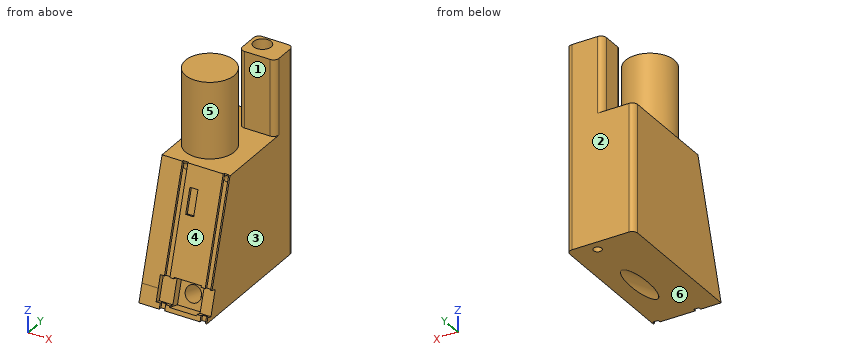
from build123d import *

# Parameters (mm, degrees)
SKETCH_1_W               = 25
SKETCH_1_H               = 60
EXTRUDE_1_DEPTH          = 75
SKETCH_3_R               = 9
CUT_EXTRUDE_1_DEPTH      = 58.142366069
SKETCH_4_R               = 3.25
CUT_EXTRUDE_2_DEPTH      = 62.320877358
SKETCH_5_R               = 1.5
CUT_EXTRUDE_3_DEPTH      = 62.320877358
SKETCH_6_W               = 25
SKETCH_6_H               = 5
CUT_EXTRUDE_4_DEPTH      = 82.738913621
CUT_EXTRUDE_5_DEPTH      = 85.557672626
SKETCH_9_R               = 3
CUT_EXTRUDE_6_DEPTH      = 85.994924721
SKETCH_10_W              = 10
SKETCH_10_H              = 10
CUT_EXTRUDE_7_DEPTH      = 5
CUT_EXTRUDE_8_DEPTH      = 15
CUT_EXTRUDE_8_DEPTH_BACK = 5
SKETCH_12_R              = 1
CUT_EXTRUDE_9_DEPTH      = 10
SKETCH_14_W              = 2
SKETCH_14_H              = 1
CUT_EXTRUDE_10_DEPTH     = 49.16
SKETCH_15_W              = 2.940527474
SKETCH_15_H              = 9
CUT_EXTRUDE_11_DEPTH     = 1
FILLET_1_R               = 2


with BuildPart() as part:
    # Эскиз1 → Бобышка-Вытянуть1 (new body)
    with BuildSketch(Plane.XY):
        Rectangle(SKETCH_1_W, SKETCH_1_H)
    extrude(amount=EXTRUDE_1_DEPTH)

    # Эскиз3 → Вырез-Вытянуть1 (cut, through all)
    with BuildSketch(Plane.XY.offset(47)):
        Polygon((-12.5, -30), (12.5, -30), (12.5, 14.25), (-1, 14.25), (-1, 30), (-12.5, 30), align=None)
        with Locations(Location((-3, 0, 0), (0, 0, 180))):
            Circle(SKETCH_3_R, mode=Mode.SUBTRACT)
    extrude(amount=CUT_EXTRUDE_1_DEPTH, mode=Mode.SUBTRACT)

    # Эскиз4 → Вырез-Вытянуть2 (cut, through all)
    with BuildSketch(Plane.XY.offset(52)):
        with Locations((3.5, 21)):
            Circle(SKETCH_4_R)
    extrude(amount=CUT_EXTRUDE_2_DEPTH, mode=Mode.SUBTRACT)

    # Эскиз5 → Вырез-Вытянуть3 (cut, through all)
    with BuildSketch(Plane.XY.offset(52)):
        with Locations((3.5, 21)):
            Circle(SKETCH_5_R)
    extrude(amount=-CUT_EXTRUDE_3_DEPTH, mode=Mode.SUBTRACT)

    # Эскиз6 → Вырез-Вытянуть4 (cut, through all)
    with BuildSketch(Plane(origin=(0, 0, 0), x_dir=(-1, 0, 0), z_dir=(0, 0, -1))):
        with Locations((0, 27.5)):
            Rectangle(SKETCH_6_W, SKETCH_6_H)
    extrude(amount=-CUT_EXTRUDE_4_DEPTH, mode=Mode.SUBTRACT)

    # Эскиз8 → Вырез-Вытянуть5 (cut, through all)
    with BuildSketch(Plane(origin=(12.5, 0, 0), x_dir=(0, 0, -1), z_dir=(1, 0, 0))):
        Polygon((-6.266839037, -25.421365839), (-47, -13.294552658), (-47, -30), (0, -30), (0, -27.287088617), align=None)
    extrude(amount=-CUT_EXTRUDE_5_DEPTH, mode=Mode.SUBTRACT)

    # Эскиз9 → Вырез-Вытянуть6 (cut, through all)
    with BuildSketch(Plane(origin=(0, -25.065453583, 7.462324694), x_dir=(1, 0, 0), z_dir=(0, -0.9584273167859609, 0.2853367807319331))):
        with Locations(Location((3.5, -1.247340968, 0), (0, 0, 270))):
            Circle(SKETCH_9_R)
    extrude(amount=-CUT_EXTRUDE_6_DEPTH, mode=Mode.SUBTRACT)

    # Эскиз10 → Вырез-Вытянуть7 (cut)
    with BuildSketch(Plane(origin=(0, -25.065453583, 7.462324694), x_dir=(1, 0, 0), z_dir=(0, -0.9584273167859609, 0.2853367807319331))):
        with Locations((3.5, -1.247340968)):
            Rectangle(SKETCH_10_W, SKETCH_10_H)
    extrude(amount=-CUT_EXTRUDE_7_DEPTH, mode=Mode.SUBTRACT)

    # Эскиз11 → Вырез-Вытянуть8 (cut, two sides: drawn at the far end of the back side and taken through both)
    with BuildSketch(Plane(origin=(-1.5, 0, 0), x_dir=(0, 0, -1), z_dir=(1, 0, 0)).offset(-CUT_EXTRUDE_8_DEPTH_BACK)):
        Polygon((-10.579761962, -24.137350326), (-1.953916111, -26.705381353), (-1.38324255, -24.788526719), (-10.009088401, -22.220495692), align=None)
    extrude(amount=CUT_EXTRUDE_8_DEPTH + CUT_EXTRUDE_8_DEPTH_BACK, mode=Mode.SUBTRACT)

    # Эскиз12 → Вырез-Вытянуть9 (cut)
    with BuildSketch(Plane(origin=(0, -25.065453583, 7.462324694), x_dir=(1, 0, 0), z_dir=(0, -0.9584273167859609, 0.2853367807319331))):
        with Locations(Location((-4, 39.752659032, 0), (0, 0, 270))):
            Circle(SKETCH_12_R)
        with Locations(Location((11, 39.752659032, 0), (0, 0, 90))):
            Circle(SKETCH_12_R)
    extrude(amount=-CUT_EXTRUDE_9_DEPTH, mode=Mode.SUBTRACT)

    # Эскиз14 → Вырез-Вытянуть10 (cut)
    with BuildSketch(Plane(origin=(0, -55.116213781, 8.285107119), x_dir=(-1, 0, 0), z_dir=(0, 0.285336780731933, 0.9584273167859609))):
        with Locations((4, -29.536239553)):
            Rectangle(SKETCH_14_W, SKETCH_14_H)
        with Locations((-11, -29.536239553)):
            Rectangle(SKETCH_14_W, SKETCH_14_H)
    extrude(amount=CUT_EXTRUDE_10_DEPTH, mode=Mode.SUBTRACT)

    # Эскиз15 → Вырез-Вытянуть11 (cut)
    with BuildSketch(Plane(origin=(0, -25.065453583, 7.462324694), x_dir=(1, 0, 0), z_dir=(0, -0.9584273167859609, 0.2853367807319331))):
        with Locations((0.529736263, 29.252659032)):
            Rectangle(SKETCH_15_W, SKETCH_15_H)
    extrude(amount=-CUT_EXTRUDE_11_DEPTH, mode=Mode.SUBTRACT)

    # Скругление1
    fillet_1_edges = [part.edges().sort_by_distance(p)[0] for p in [
        (12.5, 14.25, 61),
        (-1, 14.25, 61),
        (-1, 25, 61),
        (-12.5, 25, 23.5),
        (12.5, 25, 37.5),
    ]]
    fillet(fillet_1_edges, radius=FILLET_1_R)


solid = part.part
Read the model definition and answer for the solid it produces. Units are mm, in the model's axes. Face numbers are marked on the shaded views. A direction names the side the tool comes from. Give positions to 0.01 mm unless a question says otherwise; leave off trailing zeros. Loops run counter-clockwise (first coordinate to the right, second up) from the corner with the lowest first, then second, coordinate; pieces in that order, holes last. Notation, with made-up numbers: (-21, 64) -> (24, 64) arc R18 ccw to (24, 94) -> close; hole circle Ø8 at (-23, -24). An arc over 180 degrees is marked (long way). Answer as CSV lines item,"result".
Item 1: Find section B-B on y = 21. Give the vertices of the cut face in (x, z), plus the area to 3 significant figures.
Returned:
outline,"(-12.5, 0) -> (2, 0) -> (2, 52) -> (0.25, 52) -> (0.25, 75) -> (-1, 75) -> (-1, 47) -> (-12.5, 47) -> close; (5, 0) -> (12.5, 0) -> (12.5, 75) -> (6.75, 75) -> (6.75, 52) -> (5, 52) -> close"
area,"1,250 mm²"
Item 2: For the marked faces 5 and 6, determine the directions among +Z, -Z, +X, -X, +Y, -Y from which every point of the face is accessible in a straight line to the end or side of a thin tool.
Returned:
face 5,"+Z"
face 6,"-Z, +X, -X, +Y, -Y"
Item 3: Consider line 1 (X direction, y = 21, z = 60.75); line 2 (Y direction, x = 3.5, z = 64.25); line 3 (Y direction, x = 3.5, z = 17). Determine where each line is inside the solid, lowest interval first. Write a range as [from, to].
Returned:
line 1,"x = [-1, 0.25], [6.75, 12.5]"
line 2,"y = [-6.22, 6.22], [14.25, 17.75], [24.25, 25]"
line 3,"y = [-22.23, 19.5], [22.5, 25]"
Item 4: Find section D-D on z = 12. Give the vertices of the cut face in (x, y), plus the area to 3 significant figures.
Returned:
outline,"(-12.5, -23.71) -> (-5, -23.71) -> (-5, -22.67) -> (-3, -22.67) -> (-3, -23.71) -> (10, -23.71) -> (10, -22.67) -> (12, -22.67) -> (12, -23.71) -> (12.5, -23.71) -> (12.5, 23) arc R2 ccw to (10.5, 25) -> (-10.5, 25) arc R2 ccw to (-12.5, 23) -> close; hole circle Ø3 at (3.5, 21)"
area,"1,200 mm²"
Item 5: Find section A-A on z = 62.5. Give the vertices of the cut face in (x, y), plus the area to 3 significant figures.
Returned:
outline,"circle Ø18 at (-3, 0); (-1, 16.25) arc R2 ccw to (1, 14.25) -> (10.5, 14.25) arc R2 ccw to (12.5, 16.25) -> (12.5, 23) arc R2 ccw to (10.5, 25) -> (1, 25) arc R2 ccw to (-1, 23) -> close; hole circle Ø6.5 at (3.5, 21)"
area,"363 mm²"
Item 6: Find section C-C on x = 3.5. Give the vertices of the cut face in (y, z).
Returned:
outline,"(-27.29, 0) -> (-14.89, 0) -> (-21.49, 1.96) -> (-22.06, 0.05) -> (-26.85, 1.47) -> close; (-23.99, 11.06) -> (-19.2, 9.63) -> (-19.77, 7.72) -> (6.14, 0) -> (19.5, 0) -> (19.5, 52) -> (17.75, 52) -> (17.75, 75) -> (14.25, 75) -> (14.25, 47) -> (6.22, 47) -> (6.22, 75) -> (-6.22, 75) -> (-6.22, 47) -> (-13.29, 47) -> close; (22.5, 0) -> (25, 0) -> (25, 75) -> (24.25, 75) -> (24.25, 52) -> (22.5, 52) -> close"
Item 7: Each of these flat-tipped pins is pushed along its axis until it touches: pin 1 (5.5 mm diameter, centred on y = 18.5, z = 66, fed in from -X); pin 2 (1.8 mm diameter, centred on x = 3.5, y = 21, fed in from -Z); pin 3 (8 mm diameter, centred on x = 9.5, y = -5, fed in from -Z); pin 4 (5 mm diameter, centred on x = 5, z = 62.5, fed in from -Y). Where does it stop, or does it pass through?
Returned:
pin 1,"stops at x = -1"
pin 2,"passes through"
pin 3,"stops at z = 0"
pin 4,"stops at y = -7.12"
Item 8: Determine the mould class of the marked faces 1, 2, 3 and 4 for opening direction Y: +Y half, -Y half, draft (parallel to the pull), parting line (faces both ways), or undercut.
Returned:
face 1,"undercut"
face 2,"+Y half"
face 3,"draft"
face 4,"-Y half"
